The listing builds one solid part. Answer for the finished solid, in the listing's coordinates (mm). Coordinates: 2 decimals unless noted, no trailing zeros. Write each loop counter-clockwise with the first axis right and the second up, starting at its lowest first coordinate (ties: lowest second). Pieces come first, ordered by that corner, then holes.
(1) The part is cut by section A-A on y = 0. Determine the outline of the cut face in (x, z).
(2) For a pull along Z with two mould halves and no side action, classify faces 1 (the cylindrical face through (-0.42, 12.932, 5.362)), 2 (the cylindrical face through (-0.42, -0.07, 1.5)), 3 (the flat face through (30, 0, -3)) as +Z half, -Z half, draft (parallel to the pull), parting line (faces both ways), or undercut.
(3) The part is cut by section D-D on y = 7.25. Determine the outline of the cut face in (x, z).
(4) Given P1, Ø6, axis at x = -17.5, y = 8.5, coming from the -Z side; P2, Ø1, axis at x = -8, y = 6, coming from the +Z side; P3, Ø10, axis at x = -19, z = -11, coming from the +Y side, each flat-ended and moving along its own axis, determine where each tip first touches the part or whether it passes through.
(5) Straight lines are drawn through the part: line 1 (Z direction, x = 3, y = 0); line 2 (Z direction, x = 2.5, y = -8.75); line 3 (Y direction, x = -7, z = -4.5). For each, find the intervals that lie inside material, in ascending order.
(6) The part is cut by section C-C on x = -21. Determine the outline of the cut face in (y, z).
Autodesk Inventor part; units mm, degrees
ref_plane "YZ Plane" through (0, 0, 0) normal (1, 0, 0) x (0, 1, 0)
ref_plane "XZ Plane" through (0, 0, 0) normal (0, 1, 0) x (-1, 0, 0)
ref_plane "XY Plane" through (0, 0, 0) normal (0, 0, 1) x (1, 0, 0)
sketch "Эскиз1" plane through (0, 0, 0) normal (1, 0, 0) x (0, 1, 0)
  circle A0 centre (0, 0) radius 14
  dimension "d0" = 28
extrude "Выдавливание1" add sketch "Эскиз1" along normal mid plane 60
sketch "Эскиз2" plane through (30, 0, 0) normal (1, 0, 0) x (0, 0, -1)
  point P0 (0, 0)
  point P1 (0, 0)
hole "Отверстие1" at (30, 0, 0) direction (-1, 0, 0) diameter 3 depth 60
fillet "Сопряжение1" radius 0.1 2 edges at (-30, 0, 1.5) (30, 0, 1.5)
properties part number "Вал конвейера 2"
Model answer:
1. outline: (-30, -14) - (30, -14) - (30, -1.6) arc R0.1 ccw to (29.9, -1.5) - (-29.9, -1.5) arc R0.1 ccw to (-30, -1.6) - close; (-30, 1.6) arc R0.1 ccw to (-29.9, 1.5) - (29.9, 1.5) arc R0.1 ccw to (30, 1.6) - (30, 14) - (-30, 14) - close
2. face 1: parting line
2. face 2: undercut
2. face 3: draft
3. outline: (-30, -11.98) - (30, -11.98) - (30, 11.98) - (-30, 11.98) - close
4. P1: stops at z = -12.87
4. P2: stops at z = 12.87
4. P3: stops at y = 12.65
5. line 1: z = -14 to -1.5, 1.5 to 14
5. line 2: z = -10.93 to 10.93
5. line 3: y = -13.26 to 13.26
6. outline: circle Ø28 at (0, 0); hole circle Ø3 at (0, 0)
